Read the model definition and answer for the solid it produces. Units are mm, in the model's axes. Give positions to 0.01 mm unless a question says otherwise; leave off trailing zeros. Loops run counter-clockwise (first coordinate to the right, second up) from the corner with the lowest first, then second, coordinate; pieces in that order, holes last.
(1) Find section A-A, the plane y = 0. Write down the section's boundary in (x, z), then the cut area to 3 significant figures.
(2) Straight lines are drawn through the part: probe 1 along Y at (x, z) = (-39.5, -0.4); probe 2 along Y at (x, z) = (25, 0.05); probe 3 along Y at (x, z) = (-11, 0). For each, find the intervals that lie inside material, in ascending order.
(3) Determine the mould class of faces 1 (the face through (26.28, -52.22, -0.01)), 2 (the face through (32.136, 55.346, -0.007)), 3 (the face through (64, 0, 0)) for opening direction X: pulls with the +X half, pulls with the -X half, needs draft (parallel to the pull), parting line crosses it, or undercut.
(4) Find section B-B, the plane x = -30. Write down the section's boundary in (y, z), then the cut area to 3 significant figures.
(5) This flat-tipped pin is pushed along its axis until it touches: P1, Ø9, axis at x = 27, y = -46.77, coming from the +Z side. Where does it stop, or does it pass through?
(6) Find section C-C, the plane z = -0.1. Write down the section's boundary in (x, y) (1 decimal).
(7) Find section D-D, the plane y = -13.5. Write down the section's boundary in (x, z), then the cut area to 3 significant figures.
Autodesk Inventor part; units mm, degrees
ref_plane "YZ Plane" through (0, 0, 0) normal (1, 0, 0) x (0, 1, 0)
ref_plane "XZ Plane" through (0, 0, 0) normal (0, 1, 0) x (-1, 0, 0)
ref_plane "XY Plane" through (0, 0, 0) normal (0, 0, 1) x (1, 0, 0)
sketch "Эскиз1" plane through (0, 0, 0) normal (0, 0, 1) x (1, 0, 0)
  arc A0 (-2.1988, -43.945) -> (-9.9993, -42.8487) centre (0, 0) ccw
  arc A1 (-36.7231, 48.0765) -> (-48.1838, 38.1838) centre (-38.1838, 38.1838) ccw
  arc A2 (-36.7231, 48.0765) -> (23.0287, 55.943) centre (-20.6558, 156.8967) ccw
  arc A3 (36.9839, 47.3334) -> (23.0287, 55.943) centre (27, 46.7654) ccw
  arc A4 (36.9839, 47.3334) -> (59.4839, 8.3623) centre (86.9031, 50.1735) ccw
  arc A5 (59.4839, -8.3623) -> (59.4839, 8.3623) centre (54, 0) ccw
  arc A6 (59.4839, -8.3623) -> (36.9839, -47.3334) centre (86.9031, -50.1735) ccw
  arc A7 (25.6947, -56.6798) -> (36.9839, -47.3334) centre (27, -46.7654) ccw
  arc A8 (-48.1838, -38.1838) -> (-39.489, -48.0982) centre (-38.1838, -38.1838) ccw
  line L0 (-48.1838, 38.1838) -> (-48.1838, -38.1838)
  circle A9 centre (0, 0) radius 54 construction
  circle A10 centre (-38.1838, 38.1838) radius 5.5
  line L1 (0, 0) -> (-38.1838, 38.1838) construction
  line L2 (0, 0) -> (-54, 0) construction
  line L3 (0, 0) -> (27, 46.7654) construction
  line L4 (0, 0) -> (0, 54) construction
  circle A11 centre (27, 46.7654) radius 5.5
  circle A12 centre (54, 0) radius 5.5
  line L5 (0, 0) -> (-38.1838, -38.1838) construction
  line L6 (-39.489, -48.0982) -> (25.6947, -56.6798)
  line L7 (0, 0) -> (0, -54) construction
  line L8 (0, 0) -> (27, -46.7654) construction
  circle A13 centre (-38.1838, -38.1838) radius 5.5
  circle A14 centre (27, -46.7654) radius 5.5
  arc A15 (-46, 0) -> (0, -46) centre (0, 0) ccw construction
  line L9 (0, 0) -> (-6.402, -45.5523) construction
  arc A16 (-9.9993, -42.8487) -> (-2.1988, -43.945) centre (-6.402, -45.5523) ccw
  dimension "d4" = 108
  dimension "d0" = 88
  dimension "d1" = 10
  dimension "d2" = 110
  dimension "d3" = 50
  dimension "d5" = 11
  dimension "d6" = 45
  dimension "d7" = 30
  dimension "d8" = 90
  dimension "d9" = 30
  dimension "d10" = 46
  dimension "d11" = 8
  dimension "d12" = 4.5
extrude "Выдавливание1" add sketch "Эскиз1" along normal mid plane 1
properties part number "74. Прокладка задней крышки"
Entries:
1. outline: (-48.18, -0.5) - (-44, -0.5) - (-44, 0.5) - (-48.18, 0.5) - close; (44, -0.5) - (48.5, -0.5) - (48.5, 0.5) - (44, 0.5) - close; (59.5, -0.5) - (64, -0.5) - (64, 0.5) - (59.5, 0.5) - close
1. area: 13.2 mm2
2. probe 1: y = -48.1 to -43.52, -32.84 to -19.38, 19.38 to 32.84, 43.52 to 48.1
2. probe 2: y = -56.59 to -51.89, -41.64 to -36.21, 36.21 to 41.64, 51.89 to 56.56
2. probe 3: y = -51.85 to -42.6, 42.6 to 47.32
3. face 1: undercut
3. face 2: parting line crosses it
3. face 3: pulls with the +X half
4. outline: (-49.35, -0.5) - (-32.19, -0.5) - (-32.19, 0.5) - (-49.35, 0.5) - close; (32.19, -0.5) - (47.29, -0.5) - (47.29, 0.5) - (32.19, 0.5) - close
4. area: 32.3 mm2
5. P1: passes through
6. outline: (-48.2, -38.2) arc R10 ccw to (-39.5, -48.1) - (25.7, -56.7) arc R10 ccw to (37, -47.3) arc R50 cw to (59.5, -8.4) arc R10 ccw to (59.5, 8.4) arc R50 cw to (37, 47.3) arc R10 ccw to (23, 55.9) arc R110 cw to (-36.7, 48.1) arc R10 ccw to (-48.2, 38.2) - close; hole circle Ø11 at (-38.2, -38.2); hole circle Ø11 at (-38.2, 38.2); hole (-10, -42.8) arc R4.5 ccw (long way) to (-2.2, -43.9) arc R44 ccw (long way) to start; hole circle Ø11 at (27, -46.8); hole circle Ø11 at (27, 46.8); hole circle Ø11 at (54, 0)
7. outline: (-48.18, -0.5) - (-41.88, -0.5) - (-41.88, 0.5) - (-48.18, 0.5) - close; (41.88, -0.5) - (52.92, -0.5) - (52.92, 0.5) - (41.88, 0.5) - close
7. area: 17.3 mm2
